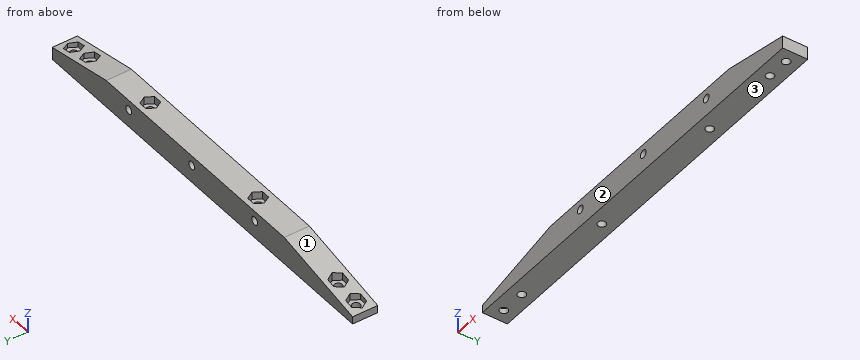
Autodesk Inventor part; units mm, degrees
ref_plane "YZ Plane" through (0, 0, 0) normal (1, 0, 0) x (0, 1, 0)
ref_plane "XZ Plane" through (0, 0, 0) normal (0, 1, 0) x (-1, 0, 0)
ref_plane "XY Plane" through (0, 0, 0) normal (0, 0, 1) x (1, 0, 0)
sketch "Sketch1" plane through (0, 0, 0) normal (0, 0, 1) x (1, 0, 0)
  line L0 (0, 0) -> (167, 0)
  line L1 (167, 0) -> (167, 10)
  line L2 (167, 10) -> (0, 10)
  line L3 (0, 10) -> (0, 0)
  circle A0 centre (59.5, 5) radius 1.6
  circle A1 centre (119.5, 5) radius 1.6
  circle A2 centre (162, 5) radius 1.6
  circle A3 centre (153, 5) radius 1.6
  circle A4 centre (15, 5) radius 1.6
  circle A5 centre (5, 5) radius 1.6
  dimension "d1" = 10
  dimension "d2" = 90
  dimension "d4" = 3.2
  dimension "d6" = 3.2
  dimension "d7" = 3.2
  dimension "d8" = 60
  dimension "d9" = 42.5
  dimension "d26" = 3.2
  dimension "d27" = 33.5
  dimension "d28" = 3.2
  dimension "d29" = 44.5
  dimension "d32" = 15
  dimension "d33" = 5
  dimension "d61" = 3.2
  dimension "d62" = 10
  dimension "d63" = 9
ref_plane "Work Plane2" through (0, 0, 0) normal (0, -1, 0) x (1, 0, 0)
sketch "Sketch2" plane through (0, 0, 0) normal (0, -1, 0) x (1, 0, 0)
  circle A0 centre (54.5, 7) radius 1.6
  circle A1 centre (124.5, 7) radius 1.6
  circle A2 centre (89.5, 7) radius 1.6
  point P0 (0, 0)
  dimension "d13" = 3.2
  dimension "d15" = 3.2
  dimension "d16" = 70
  dimension "d17" = 3.2
  dimension "d18" = 35
  dimension "d64" = 54.5
  dimension "d65" = 35
ref_plane "Work Plane1" through (0, 0, 11) normal (0, 0, 1) x (1, 0, 0)
extrude "klocek" add sketch "Sketch1" along normal blind 11
ref_plane "Work Plane3" through (0, 0, 0) normal (0, -1, 0) x (1, 0, 0)
extrude "prowadzenie osi" cut sketch "Sketch2" against normal up to next
ref_plane "Work Plane4" through (0, 0, 0) normal (0, -1, 0) x (1, 0, 0)
sketch "Sketch7" plane through (0, 0, 0) normal (0, -1, 0) x (1, 0, 0)
  line L0 (0, 11) -> (0, 3)
  line L1 (0, 11) -> (167, 11)
  line L2 (0, 11) -> (38, 11)
  line L3 (38, 11) -> (0, 3)
  point P0 (0, -1.8333)
  dimension "d86" = 8
  dimension "d87" = 38
sketch "Sketch8" plane through (0, 0, 0) normal (0, -1, 0) x (1, 0, 0)
  line L0 (167, 0) -> (167, 11)
  line L1 (167, 11) -> (167, 5)
  line L2 (167, 11) -> (0, 11)
  line L3 (167, 11) -> (137, 11)
  line L4 (137, 11) -> (167, 5)
  point P0 (0, 0)
  point P1 (40.8333, 11)
  dimension "d80" = 6
  dimension "d81" = 30
extrude "przedni skos" cut sketch "Sketch7" against normal up to next
extrude "tylni skos" cut sketch "Sketch8" against normal up to next
ref_plane "Work Plane7" through (0, 0, 11) normal (0, 0, 1) x (1, 0, 0)
sketch "Sketch5" plane through (0, 0, 11) normal (0, 0, 1) x (1, 0, 0)
  line L0 (62.9064, 5) -> (61.2032, 2.05)
  line L1 (61.2032, 2.05) -> (57.7968, 2.05)
  line L2 (57.7968, 2.05) -> (56.0936, 5)
  line L3 (56.0936, 5) -> (57.7968, 7.95)
  line L4 (57.7968, 7.95) -> (61.2032, 7.95)
  line L5 (61.2032, 7.95) -> (62.9064, 5)
  line L6 (122.9064, 5) -> (121.2032, 2.05)
  line L7 (121.2032, 2.05) -> (117.7968, 2.05)
  line L8 (117.7968, 2.05) -> (116.0936, 5)
  line L9 (116.0936, 5) -> (117.7968, 7.95)
  line L10 (117.7968, 7.95) -> (121.2032, 7.95)
  line L11 (121.2032, 7.95) -> (122.9064, 5)
  point P0 (59.5, 5)
  point P1 (119.5, 5)
  point P2 (119.5, 5)
  dimension "d44" = 5.9
  dimension "d45" = 5.9
extrude "hex insert middle" cut sketch "Sketch5" against normal blind 3
ref_plane "Work Plane6" through (0, 0, 11) normal (0, 0, 1) x (1, 0, 0)
sketch "Sketch9" plane through (0, 0, 11) normal (0, 0, 1) x (1, 0, 0)
  line L0 (156.4064, 5) -> (154.7032, 2.05)
  line L1 (154.7032, 2.05) -> (151.2968, 2.05)
  line L2 (151.2968, 2.05) -> (149.5936, 5)
  line L3 (149.5936, 5) -> (151.2968, 7.95)
  line L4 (151.2968, 7.95) -> (154.7032, 7.95)
  line L5 (154.7032, 7.95) -> (156.4064, 5)
  point P0 (0, 0)
  point P1 (153, 5)
  point P2 (153, 5)
  dimension "d51" = 5.9
extrude "hex insert rear 1" cut sketch "Sketch9" against normal blind 6
ref_plane "Work Plane5" through (0, 0, 11) normal (0, 0, 1) x (1, 0, 0)
sketch "Sketch10" plane through (0, 0, 11) normal (0, 0, 1) x (1, 0, 0)
  line L0 (160.2968, 7.95) -> (163.7032, 7.95)
  line L1 (163.7032, 7.95) -> (165.4064, 5)
  line L2 (165.4064, 5) -> (163.7032, 2.05)
  line L3 (163.7032, 2.05) -> (160.2968, 2.05)
  line L4 (160.2968, 2.05) -> (158.5936, 5)
  line L5 (158.5936, 5) -> (160.2968, 7.95)
  point P0 (0, 0)
  point P1 (162, 5)
  point P2 (162, 5)
  dimension "d72" = 5.9
extrude "hex insert rear 2" cut sketch "Sketch10" against normal blind 7.5
sketch "Sketch13" plane through (0, 0, 11) normal (0, 0, 1) x (1, 0, 0)
  circle A0 centre (5, 5) radius 1.6
  line L0 (8.4064, 5) -> (6.7032, 2.05)
  line L1 (6.7032, 2.05) -> (3.2968, 2.05)
  line L2 (3.2968, 2.05) -> (1.5936, 5)
  line L3 (1.5936, 5) -> (3.2968, 7.95)
  line L4 (3.2968, 7.95) -> (6.7032, 7.95)
  line L5 (6.7032, 7.95) -> (8.4064, 5)
  point P0 (0, 0)
  dimension "d90" = 5.9
extrude "Extrusion18" cut sketch "Sketch13" against normal blind 9
sketch "Sketch16" plane through (0, 0, 11) normal (0, 0, 1) x (1, 0, 0)
  circle A0 centre (15, 5) radius 1.6
  line L0 (18.4064, 5) -> (16.7032, 2.05)
  line L1 (16.7032, 2.05) -> (13.2968, 2.05)
  line L2 (13.2968, 2.05) -> (11.5936, 5)
  line L3 (11.5936, 5) -> (13.2968, 7.95)
  line L4 (13.2968, 7.95) -> (16.7032, 7.95)
  line L5 (16.7032, 7.95) -> (18.4064, 5)
  point P0 (0, 0)
  dimension "d93" = 5.9
extrude "Extrusion19" cut sketch "Sketch16" against normal blind 7.5
properties part number "new_wheel_support_v3"
For this review, take the finished solid that the model builds, in its own axes (mm). Face numbers are marked on the shaded views. Round coordinates to 2 decimals unless told otherwise and drop trailing zeros. Order: outer loops, then holes, each group sorted by start corner. A loop starts at its lowest first (then second) coordinate and runs counter-clockwise, first axis right, second up. Notation, with made-up numbers: M 13,67 L 71,67 A20 cw 71,98 Z; hole C -22,83 d2. An arc over 180 degrees is marked long. Write each question's results on one line, items separated by ' | '. Start each with the question number.
1. Draft analysis for pull direction Z (two halves, no side actions). For the marked faces 1, 2 and 3, state which applies: pulls with the +Z half, pulls with the -Z half, needs draft (parallel to the pull), parting line crosses it, or undercut.
2. To check wall thickness, follow L1, parallel to Z at x = 124.5, y = 3.5; L2, parallel to Y at x = 153, z = 2.1; L3, parallel to Z at x = 116.5, y = 5. State the ranges of each line that lie inside material, in increasing order. Write a range as [from, to].
3. Add section C-C (x = 15). State the section outline as (y, z) points.
4. Add section A-A (x = 124.5). State the section outline as (y, z) points, then the cut area to 3 significant figures.
5. Clearance check with flat-ended pins moving along their axes: pin 1 Ø3 at (x, y) = (61, 5) entering from +Z; pin 2 Ø4.5 at (x, y) = (15.5, 6) entering from +Z. State where each tip first meets the part, or that it passes through.
6. Add section B-B (x = 162). State the section outline as (y, z) points.
Output values:
1) face 1: pulls with the +Z half | face 2: needs draft | face 3: pulls with the -Z half
2) L1: [0, 5.4], [8.6, 11] | L2: [0, 3.4], [6.6, 10] | L3: [0, 8]
3) outline: M 0,0 L 3.4,0 L 3.4,3.5 L 2.05,3.5 L 2.05,6.16 L 0,6.16 Z; M 6.6,0 L 10,0 L 10,6.16 L 7.95,6.16 L 7.95,3.5 L 6.6,3.5 Z
4) outline: M 0,0 L 10,0 L 10,5.4 L 0,5.4 Z; M 0,8.6 L 10,8.6 L 10,11 L 0,11 Z | area: 78.0 mm^2
5) pin 1: z = 8 | pin 2: z = 6.74
6) outline: M 0,0 L 3.4,0 L 3.4,3.5 L 2.05,3.5 L 2.05,6 L 0,6 Z; M 6.6,0 L 10,0 L 10,6 L 7.95,6 L 7.95,3.5 L 6.6,3.5 Z
